Geometry: final body of the model. Coordinates: model frame, mm. A direction names the side the tool comes from. Give positions to 0.01 mm unless a question says otherwise; leave off trailing zeros. Loops run counter-clockwise (first coordinate to the right, second up) from the corner with the lowest first, then second, coordinate; pieces in that order, holes last. Notation, with made-up numbers: (11, 48) -> (70, 48) arc R23 cw to (70, 63) -> close; hole circle Ø4 at (21, 1). An arc over 180 degrees is marked (long way). Answer in a Markdown table with one row per item. Add a question column.
1) First-contact query: P1, Ø11, axis at x = 7, z = -2.5, coming from the -Y side (3 decimals); P2, Ø12, axis at y = 4, z = -18.5, coming from the -X side; P3, Ø4, axis at x = 1, z = -12.5, coming from the +Y side. Flat tips, straight axial feed; report the tip coordinate or a pass-through.
2) Section query D-D (y = 14.5). Return the cut outline in (x, z) (1 decimal), plus the area to 3 significant figures.
3) Access query for faces 1 (the flat face through (10.033, 2, -44)), 2 (the flat face through (5.906, 15, -37)), 3 (the flat face through (0, 4, 26.67)). Directions: +Z, -Z, +X, -X, +Y, -Y. A direction counts if a zero-diameter tool reaches every point of the face in a straight line with its end or side. Return the directions, or none.
4) Section query C-C (x = -4). Return the cut outline in (y, z) (3 decimals).
5) Draft query along Z for faces 4 (the flat face through (-9, 15, 31.115)), 5 (the flat face through (-2.54, 22, 0)), 6 (the flat face through (0, 0, 38)). Return one class per face: +Z half, -Z half, draft (parallel to the pull), parting line (faces both ways), or undercut.
6) Line query: line 1 (Z direction, x = 10.5, y = 6.75) (3 decimals); line 2 (Z direction, x = -2.5, y = 6.25); line 3 (Z direction, x = 10, y = 17) (3 decimals). Output: solid intervals per line, ascending. Write a range as from..to.
7) Section query B-B (z = 1.5). Return the cut outline in (x, y) (3 decimals), plus the area to 3 significant figures.
8) Section query A-A (y = 3.5). Give the number of separate pieces and of enclosed holes in the cut face, plus the area to 3 significant figures.
Autodesk Inventor part; units mm, degrees
ref_plane "YZ Plane" through (0, 0, 0) normal (1, 0, 0) x (0, 1, 0)
ref_plane "XZ Plane" through (0, 0, 0) normal (0, 1, 0) x (-1, 0, 0)
ref_plane "XY Plane" through (0, 0, 0) normal (0, 0, 1) x (1, 0, 0)
sketch "Sketch1" plane through (0, 0, 0) normal (0, 1, 0) x (-1, 0, 0)
  line L0 (-15.875, 49.53) -> (15.875, 49.53)
  line L1 (15.875, 49.53) -> (15.875, -49.53)
  line L2 (15.875, -49.53) -> (-15.875, -49.53)
  line L3 (-15.875, -49.53) -> (-15.875, 49.53)
  line L4 (-15.875, 49.53) -> (15.875, -49.53) construction
  line L5 (15.875, 49.53) -> (-15.875, -49.53) construction
  line L6 (15.875, -49.53) -> (15.875, -48.26)
  line L7 (15.875, -49.53) -> (17.145, -49.53) construction
  line L8 (15.875, 49.53) -> (15.875, 48.26)
  line L9 (15.875, 49.53) -> (17.145, 49.53) construction
  line L10 (15.875, -49.53) -> (14.097, -49.53)
  line L11 (-15.875, -49.53) -> (-14.097, -49.53)
  line L12 (15.875, -49.53) -> (15.875, -39.37)
  line L13 (15.875, 49.53) -> (15.875, 39.37)
  line L14 (14.097, 49.53) -> (12.065, 49.53)
  line L15 (-14.097, 49.53) -> (-12.065, 49.53)
  line L16 (-12.065, -39.37) -> (-12.065, -48.26) construction
  line L17 (-10.033, -41.402) -> (-10.033, -46.228)
  line L18 (-14.097, -46.228) -> (-14.097, -41.402)
  arc A0 (-10.033, -41.402) -> (-14.097, -41.402) centre (-12.065, -41.402) ccw
  arc A1 (-14.097, -46.228) -> (-10.033, -46.228) centre (-12.065, -46.228) ccw
  line L19 (12.065, -48.26) -> (12.065, -39.37) construction
  line L20 (10.033, -46.228) -> (10.033, -41.402)
  line L21 (14.097, -41.402) -> (14.097, -46.228)
  arc A2 (10.033, -46.228) -> (14.097, -46.228) centre (12.065, -46.228) ccw
  arc A3 (14.097, -41.402) -> (10.033, -41.402) centre (12.065, -41.402) ccw
  line L22 (12.065, 39.37) -> (12.065, 48.26) construction
  line L23 (10.033, 41.402) -> (10.033, 46.228)
  line L24 (14.097, 46.228) -> (14.097, 41.402)
  arc A4 (10.033, 41.402) -> (14.097, 41.402) centre (12.065, 41.402) ccw
  arc A5 (14.097, 46.228) -> (10.033, 46.228) centre (12.065, 46.228) ccw
  line L25 (-12.065, 39.37) -> (-12.065, 48.26) construction
  line L26 (-10.033, 41.402) -> (-10.033, 46.228)
  line L27 (-14.097, 46.228) -> (-14.097, 41.402)
  arc A6 (-14.097, 41.402) -> (-10.033, 41.402) centre (-12.065, 41.402) ccw
  arc A7 (-10.033, 46.228) -> (-14.097, 46.228) centre (-12.065, 46.228) ccw
  line L28 (-12.065, 49.53) -> (-12.065, 37.6428)
  line L29 (-12.065, -37.6428) -> (-12.065, -49.53)
  line L30 (-14.097, -49.53) -> (-14.097, -39.37)
  line L31 (-14.097, 39.37) -> (-14.097, 49.53)
  line L32 (12.065, 49.53) -> (12.065, 37.6428)
  line L33 (12.065, -37.6428) -> (12.065, -49.53)
  line L34 (14.097, -49.53) -> (14.097, -39.37)
  line L35 (14.097, 39.37) -> (14.097, 49.53)
  line L36 (15.875, 39.37) -> (12.065, 39.37)
  line L37 (-12.065, 39.37) -> (-15.875, 39.37)
  line L38 (15.875, 48.26) -> (12.065, 48.26)
  line L39 (-12.065, 48.26) -> (-15.875, 48.26)
  line L40 (15.875, -39.37) -> (12.065, -39.37)
  line L41 (-12.065, -39.37) -> (-15.875, -39.37)
  line L42 (15.875, -48.26) -> (12.065, -48.26)
  line L43 (-12.065, -48.26) -> (-15.875, -48.26)
  point P0 (0, 0)
  point P1 (-12.065, -43.815)
  point P2 (12.065, -43.815)
  point P3 (12.065, 43.815)
  point P4 (-12.065, 43.815)
  dimension "d0" = 31.75
  dimension "d1" = 99.06
  dimension "d2" = 1.27
  dimension "d3" = 90
  dimension "d4" = 1.27
  dimension "d5" = 90
  dimension "d6" = 1.778
  dimension "d8" = 1.778
  dimension "d10" = 10.16
  dimension "d11" = 10.16
  dimension "d12" = 2.032
  dimension "d13" = 2.032
extrude "Extrusion1" add sketch "Sketch1" along normal blind 4.445 contours L0 L31 L39 L3 | L0 L28 L39 L31 | L39 L31 L27 L37 L3 | L0 L32 A5 L23 A4 L36 L1 L40 A3 L20 A2 L33 L2 L29 A1 L17 A0 L41 L3 L37 A6 L26 A7 L28 | L39 A7 L31 | L0 L35 L38 L32 | L41 L30 L18 L43 L3 | L31 A6 L37 | L0 L1 L38 L35 | L38 L35 A5 | L43 L30 L2 L3 | L41 A0 L30 | L38 L1 L36 L35 L24 | A4 L35 L36 | L43 L29 L2 L30 | L30 A1 L43 | L1 L42 L34 L21 L40 | L33 L42 L34 L2 | L1 L2 L34 L42 | L34 A3 L40 | A2 L34 L42
sketch "Sketch2" plane through (0, 4.445, 0) normal (0, 1, 0) x (1, 0, 0)
  line L0 (15.875, -49.53) -> (15.875, 49.53)
  line L1 (-15.875, -31.115) -> (15.875, -31.115)
  line L2 (15.875, -31.115) -> (15.875, 31.115)
  line L3 (15.875, 31.115) -> (-15.875, 31.115)
  line L4 (-15.875, 31.115) -> (-15.875, -31.115)
  line L5 (-15.875, -31.115) -> (15.875, 31.115) construction
  line L6 (15.875, -31.115) -> (-15.875, 31.115) construction
  line L7 (-12.7, -31.115) -> (12.7, -31.115)
  line L8 (12.7, -31.115) -> (12.7, 31.115)
  line L9 (12.7, 31.115) -> (-12.7, 31.115)
  line L10 (-12.7, 31.115) -> (-12.7, -31.115)
  line L11 (-12.7, -31.115) -> (12.7, 31.115) construction
  line L12 (12.7, -31.115) -> (-12.7, 31.115) construction
  line L13 (-12.7, -26.67) -> (12.7, -26.67)
  line L14 (12.7, -26.67) -> (12.7, 26.67)
  line L15 (12.7, 26.67) -> (-12.7, 26.67)
  line L16 (-12.7, 26.67) -> (-12.7, -26.67)
  line L17 (-12.7, -26.67) -> (12.7, 26.67) construction
  line L18 (12.7, -26.67) -> (-12.7, 26.67) construction
  point P0 (0, 0)
  dimension "d16" = 62.23
  dimension "d19" = 25.4
  dimension "d20" = 53.34
extrude "Extrusion2" cut sketch "Sketch2" against normal blind 4.445 contours L1 L8 L3 L0 | L1 L4 L3 L10 | L13 L10 L15 L8
sketch "Sketch3" plane through (0, 4.445, 0) normal (0, 1, 0) x (1, 0, 0)
  line L0 (12.7, 31.115) -> (12.7, 26.67)
  line L1 (-12.7, -31.115) -> (12.7, -31.115)
  line L2 (12.7, -31.115) -> (12.7, 31.115)
  line L3 (12.7, 31.115) -> (-12.7, 31.115)
  line L4 (-12.7, 31.115) -> (-12.7, -31.115)
  line L5 (-12.7, -31.115) -> (12.7, 31.115) construction
  line L6 (12.7, -31.115) -> (-12.7, 31.115) construction
  line L7 (15.875, 49.53) -> (-15.875, 49.53)
  line L8 (0, 49.53) -> (0, -49.53)
  line L9 (-15.875, -49.53) -> (15.875, -49.53)
  line L10 (0, 26.67) -> (0, 34.925)
  line L11 (12.7, -26.67) -> (-12.7, -26.67)
  line L12 (0, -26.67) -> (0, -34.925)
  line L13 (-12.7, 26.67) -> (12.7, 26.67)
  line L14 (-5.9055, 43.18) -> (5.9055, 43.18)
  line L15 (5.9055, 43.18) -> (5.9055, 26.67)
  line L16 (5.9055, 26.67) -> (-5.9055, 26.67)
  line L17 (-5.9055, 26.67) -> (-5.9055, 43.18)
  line L18 (-5.9055, 43.18) -> (5.9055, 26.67) construction
  line L19 (5.9055, 43.18) -> (-5.9055, 26.67) construction
  line L20 (-5.9055, -43.18) -> (5.9055, -43.18)
  line L21 (5.9055, -43.18) -> (5.9055, -26.67)
  line L22 (5.9055, -26.67) -> (-5.9055, -26.67)
  line L23 (-5.9055, -26.67) -> (-5.9055, -43.18)
  line L24 (-5.9055, -43.18) -> (5.9055, -26.67) construction
  line L25 (5.9055, -43.18) -> (-5.9055, -26.67) construction
  point P0 (0, 0)
  point P1 (-5.9055, -31.115)
  point P2 (5.9055, -31.115)
  point P3 (-5.9055, 31.115)
  point P4 (5.9055, 31.115)
  dimension "d23" = 8.255
  dimension "d24" = 8.255
  dimension "d25" = 11.811
extrude "Extrusion3" add sketch "Sketch3" along normal blind 20.955
sketch "Sketch4" plane through (0, 25.4, 0) normal (0, 1, 0) x (1, 0, 0)
  line L0 (12.7, -26.67) -> (-12.7, -26.67)
  line L1 (-12.7, 26.67) -> (12.7, 26.67)
  line L2 (12.7, 26.67) -> (12.7, -26.67)
  line L3 (12.7, -26.67) -> (-12.7, -26.67)
  line L4 (-12.7, -26.67) -> (-12.7, 26.67)
  line L5 (-12.7, 26.67) -> (12.7, -26.67) construction
  line L6 (12.7, 26.67) -> (-12.7, -26.67) construction
  point P0 (0, 0)
extrude "Extrusion4" cut sketch "Sketch4" against normal blind 2.54
sketch "Sketch5" plane through (0, 22.86, 0) normal (0, 1, 0) x (1, 0, 0)
  line L0 (12.7, -26.67) -> (12.7, 26.67)
  line L1 (-12.7, 26.67) -> (12.7, 26.67)
  line L2 (12.7, 26.67) -> (12.7, -26.67)
  line L3 (12.7, -26.67) -> (-12.7, -26.67)
  line L4 (-12.7, -26.67) -> (-12.7, 26.67)
  line L5 (-12.7, 26.67) -> (12.7, -26.67) construction
  line L6 (12.7, 26.67) -> (-12.7, -26.67) construction
  line L7 (-2.54, 26.67) -> (2.54, 26.67)
  line L8 (2.54, 26.67) -> (2.54, -26.67)
  line L9 (2.54, -26.67) -> (-2.54, -26.67)
  line L10 (-2.54, -26.67) -> (-2.54, 26.67)
  line L11 (-2.54, 26.67) -> (2.54, -26.67) construction
  line L12 (2.54, 26.67) -> (-2.54, -26.67) construction
  point P0 (0, 0)
  dimension "d28" = 5.08
extrude "Extrusion5" cut sketch "Sketch5" against normal blind 2.54 contours L3 L8 L1 L0 | L3 L4 L1 L10
sketch "Sketch6" plane through (0, 4.445, 0) normal (0, -1, 0) x (1, 0, 0)
  line L0 (12.7, -26.67) -> (12.7, 26.67)
  line L1 (-12.7, 26.67) -> (12.7, 26.67)
  line L2 (12.7, 26.67) -> (12.7, -26.67)
  line L3 (12.7, -26.67) -> (-12.7, -26.67)
  line L4 (-12.7, -26.67) -> (-12.7, 26.67)
  line L5 (-12.7, 26.67) -> (12.7, -26.67) construction
  line L6 (12.7, 26.67) -> (-12.7, -26.67) construction
  line L7 (-2.54, 26.67) -> (2.54, 26.67)
  line L8 (2.54, 26.67) -> (2.54, -26.67)
  line L9 (2.54, -26.67) -> (-2.54, -26.67)
  line L10 (-2.54, -26.67) -> (-2.54, 26.67)
  line L11 (-2.54, 26.67) -> (2.54, -26.67) construction
  line L12 (2.54, 26.67) -> (-2.54, -26.67) construction
  point P0 (0, 0)
  dimension "d31" = 5.08
extrude "Extrusion6" cut sketch "Sketch6" against normal blind 2.54 contours L3 L8 L1 L0 | L3 L4 L1 L10
equation "\"d17\" = d14"
properties part number "12v_heater_mount"
Evaluation:
| question | item | result |
|---|---|---|
| 1 | P1 | y = 4.445 |
| 1 | P2 | x = -12.7 |
| 1 | P3 | y = 22.86 |
| 2 | outline | (-12.7, -31.1) -> (-5.9, -31.1) -> (-5.9, -43.2) -> (5.9, -43.2) -> (5.9, -31.1) -> (12.7, -31.1) -> (12.7, 31.1) -> (5.9, 31.1) -> (5.9, 43.2) -> (-5.9, 43.2) -> (-5.9, 31.1) -> (-12.7, 31.1) -> close |
| 2 | area | 1,870 mm² |
| 3 | face 1 | +Y, -Y |
| 3 | face 2 | -Z, +X, +Y |
| 3 | face 3 | -Y |
| 4 | outline | (0, -49.53) -> (4.445, -49.53) -> (4.445, -43.18) -> (25.4, -43.18) -> (25.4, -26.67) -> (20.32, -26.67) -> (20.32, 26.67) -> (25.4, 26.67) -> (25.4, 43.18) -> (4.445, 43.18) -> (4.445, 49.53) -> (0, 49.53) -> (0, 26.67) -> (6.985, 26.67) -> (6.985, -26.67) -> (0, -26.67) -> close |
| 5 | face 4 | +Z half |
| 5 | face 5 | undercut |
| 5 | face 6 | draft |
| 6 | line 1 | -31.115..-26.67, 26.67..31.115 |
| 6 | line 2 | -43.18..43.18 |
| 6 | line 3 | -31.115..31.115 |
| 7 | outline | (-12.7, 6.985) -> (-2.54, 6.985) -> (-2.54, 4.445) -> (2.54, 4.445) -> (2.54, 6.985) -> (12.7, 6.985) -> (12.7, 20.32) -> (2.54, 20.32) -> (2.54, 22.86) -> (-2.54, 22.86) -> (-2.54, 20.32) -> (-12.7, 20.32) -> close |
| 7 | area | 365 mm² |
| 8 | separate pieces | 2 |
| 8 | enclosed holes | 4 |
| 8 | area | 1,260 mm² |
